```python
from build123d import *

# Parameters (mm, degrees)
EXTRUDE_388_DEPTH = 6.4
FILLET_1259_R     = 0.4


with BuildPart() as part:
    # 草图1 → Extrude 388 (new body)
    with BuildSketch(Plane(origin=(0, 0, 0), x_dir=(0, 0, -1), z_dir=(1, 0, 0))):
        Polygon((8, 4.618802154), (8, -4.618802154), (0, -9.237604307), (-8, -4.618802154), (-8, 4.618802154), (0, 9.237604307), align=None)
    extrude(amount=EXTRUDE_388_DEPTH)

    # 草图2 → 凸台-旋转1 (revolve)
    with BuildSketch(Plane.XY, mode=Mode.PRIVATE) as revolve_1_sk:
        Polygon((0, 0), (31.4, 0), (31.4, 3.701), (31.4, 5), (0, 5), align=None)
    revolve(revolve_1_sk.sketch.rotate(Axis((0, 0, 0), (1, 0, 0)), 90), axis=Axis((0, 0, 0), (1, 0, 0)))

    # 草图3 → 切除-旋转1 (revolve, cut)
    with BuildSketch(Plane.XY):
        Polygon((0, 8), (3.601282526, 14.237604307), (3.601282526, 19.237604307), (-10, 19.237604307), (-10, 8), align=None)
    revolve(axis=Axis((0, 0, 0), (1, 0, 0)), mode=Mode.SUBTRACT)

    # 草图4 → 切除-旋转3 (revolve, cut)
    with BuildSketch(Plane.XY, mode=Mode.PRIVATE) as cut_revolve_3_sk:
        Polygon((6.4, 7.315), (5.8, 7.661410162), (5.8, 9.237604307), (6.4, 9.237604307), align=None)
    revolve(cut_revolve_3_sk.sketch.rotate(Axis((0, 0, 0), (1, 0, 0)), 90), axis=Axis((0, 0, 0), (1, 0, 0)), mode=Mode.SUBTRACT)

    # Fillet 1259
    fillet_1259_edges = [part.edges().sort_by_distance(p)[0] for p in [
        (6.4, 0, -5),
    ]]
    fillet(fillet_1259_edges, radius=FILLET_1259_R)

    # 草图6 → 切除-旋转4 (revolve, cut)
    with BuildSketch(Plane.XY, mode=Mode.PRIVATE) as cut_revolve_4_sk:
        Polygon((30.65, 5), (32.15, 5), (31.4, 3.700961894), align=None)
    revolve(cut_revolve_4_sk.sketch.rotate(Axis((0, 0, 0), (1, 0, 0)), 90), axis=Axis((0, 0, 0), (1, 0, 0)), mode=Mode.SUBTRACT)


solid = part.part
```
For this review, take the finished solid that the model builds, in its own axes (mm). A direction names the side the tool comes from. Give positions to 0.01 mm unless a question says otherwise; leave off trailing zeros. Write each loop counter-clockwise with the first axis right and the second up, starting at its lowest first coordinate (ties: lowest second). Pieces come first, ordered by that corner, then holes.
Item 1: Machinability: for faces 1 (the face through (2.859, 6.961, -3.944)), 2 (the face through (19, 0, -5)), which of the approach directions +Z, -Z, +X, -X, +Y, -Y give a long, thin tool a straight path to every point of the face, cutting with its end or side? Answer none if there is none.
Item 2: Insertion check: P1, Ø2, axis at y = 7, z = 4, coming from the -X side; P2, Ø8, axis at x = 20, z = 5.5, coming from the +Y side; P3, Ø2, axis at x = 7, z = 1.5, coming from the +Y side; P4, Ø8, axis at x = 13, y = -5.5, coming from the +Z side. Each pin has a flat end and moves straight along its axis. Give the tip position at first contact, or say it passes through.
Item 3: Wall thickness on probe 1 along Z at (x, y) = (14, 3); probe 2 along X at (y, z) = (-7.75, 1.5); probe 3 along X at (y, z) = (-6.5, -1.25): over which ranges is each line inside the solid? List them lowest first.
Item 4: Take a section at B-B (x = 29). Give the boundary of the cut face in (y, z), and give its area (3 significant figures).
Item 5: Take a section at A-A (x = 5). Give the boundary of the cut face in (y, z), and give its area (3 significant figures).
Established:
1. face 1: -Z, +X, -X, +Y
1. face 2: +X
2. P1: stops at x = 0
2. P2: stops at y = 4.77
2. P3: stops at y = 7.42
2. P4: stops at z = 4.77
3. probe 1: z = -4 to 4
3. probe 2: x = 0 to 5.8
3. probe 3: x = 0 to 6.4
4. outline: circle Ø10 at (0, 0)
4. area: 78.5 mm2
5. outline: (-9.24, 0) - (-4.62, -8) - (4.62, -8) - (9.24, 0) - (4.62, 8) - (-4.62, 8) - close
5. area: 222 mm2
